Can you work these out from the drawing? Everything is in mm from the part's minimum corner. A direction names the side the tool comes from. Round coordinates to 2 decimals unless told otherwise and drop trailing zeros. Order: outer loops, then holes, each group sorted by start corner. A loop starts at its lowest first (then second) coordinate and runs counter-clockwise, first axis right, second up. Notation, with made-up numbers: M -13.5,-12.5 L 20.5,-12.5 A23 cw 20.5,20.5 Z; hole C 66.25,87.25 d5. An arc over 180 degrees is marked long. Write item = value, one per line. Start each with the question number.
Item 1: We'd pull the mould along X, two halves only. Please class the marked faces 3, 4 and 5: pulls with the +X half, pulls with the -X half, needs draft (parallel to the pull), parting line crosses it, or undercut.
Item 2: I want a section at C-C, the plane x = 33.5. List the corners of the cut face in (y, z) for me (3 decimals), plus the area to 3 significant figures.
Item 3: I want a section at B-B, the plane y = 73. List the corners of the cut face in (x, z) for me (3 decimals).
Item 4: I'm going to push a flat-ended pin straight in: P1, Ø12, axis at x = 58, y = 27.5, coming from the -Z side. Where does the tip first touch, or does it pass through?
Item 5: Please list where these lines run through material, in increasing order: L1, parallel to X at y = 27.5, z = 35 (3 decimals); L2, parallel to Y at x = 25.5, z = 7.5 (3 decimals); L3, parallel to Z at x = 72, y = 20.
Item 6: For the marked faces 1 and 2, which set-ups out of +Z, -Z, +X, -X, +Y, -Y let a thin tool reach every point of the face, with its end or its side?
Item 7: I want a section at A-A, the plane z = 52.5. List the corners of the cut face in (x, y) for me (3 decimals), plus the area to 3 significant figures.
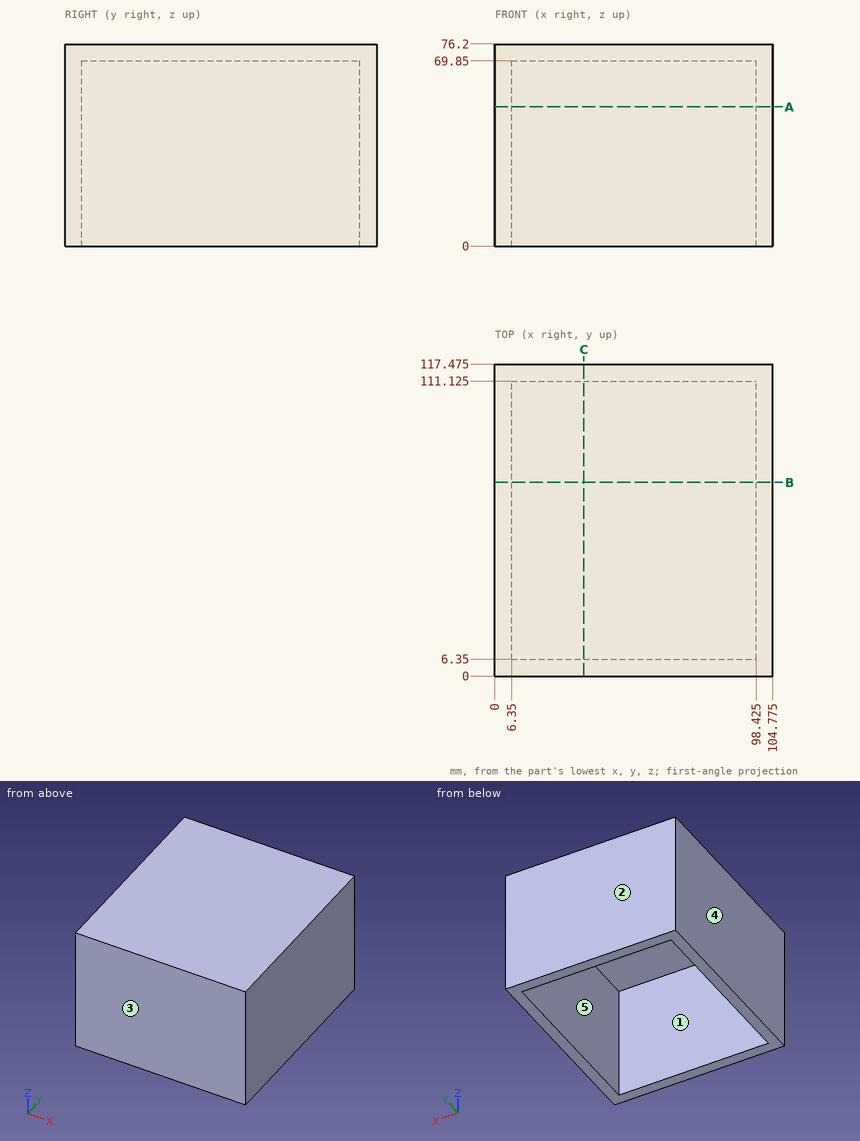
Filled in:
q1.face_3 = needs draft
q1.face_4 = pulls with the -X half
q1.face_5 = undercut
q2.outline = M 0,0 L 6.35,0 L 6.35,69.85 L 111.125,69.85 L 111.125,0 L 117.475,0 L 117.475,76.2 L 0,76.2 Z
q2.area = 1,630 mm^2
q3.outline = M 0,0 L 6.35,0 L 6.35,69.85 L 98.425,69.85 L 98.425,0 L 104.775,0 L 104.775,76.2 L 0,76.2 Z
q4.P1 = 69.85
q5.L1 = 0 to 6.35, 98.425 to 104.775
q5.L2 = 0 to 6.35, 111.125 to 117.475
q5.L3 = 69.85 to 76.2
q6.face_1 = -Z
q6.face_2 = +Z, -Z, +X, -X, +Y
q7.outline = M 0,0 L 104.775,0 L 104.775,117.475 L 0,117.475 Z; hole M 6.35,6.35 L 98.425,6.35 L 98.425,111.125 L 6.35,111.125 Z
q7.area = 2,660 mm^2
